from build123d import *

# Parameters (mm, degrees)
SKETCH1_W                 = 72.58
SKETCH1_H                 = 57.34
SKETCH1_R                 = 1.5
BOSS_EXTRUDE1_DEPTH       = 4.1
SKETCH2_W                 = 72.58
SKETCH2_H                 = 57.34
SKETCH2_R                 = 1.5
BOSS_EXTRUDE2_DEPTH       = 0.5
SKETCH2_4_W               = 72.58
SKETCH2_4_H               = 57.34
SKETCH2_4_R               = 1.5
BOSS_EXTRUDE3_DEPTH       = 4
BOSS_EXTRUDE4_START       = 4
BOSS_EXTRUDE4_OUTLINE_W   = 72.58
BOSS_EXTRUDE4_OUTLINE_H   = 57.34
BOSS_EXTRUDE4_OUTLINE_W_2 = 68.58
BOSS_EXTRUDE4_OUTLINE_H_2 = 53.34
BOSS_EXTRUDE4_DEPTH       = 1.5
SKETCH4_W                 = 70.58
SKETCH4_H                 = 55.34
SKETCH4_W_2               = 68.58
SKETCH4_H_2               = 53.34
BOSS_EXTRUDE5_DEPTH       = 10
FILLET1_R                 = 1
FILLET2_R                 = 0.5
FILLET3_R                 = 0.75
SKETCH3_W                 = 36.5
SKETCH3_H                 = 36.5
CUT_EXTRUDE1_DEPTH        = 51.230399162
SKETCH6_W                 = 11
SKETCH6_H                 = 12
SKETCH6_W_2               = 13.6
SKETCH6_H_2               = 13.6
CUT_EXTRUDE2_DEPTH        = 3
CHAMFER1_SIZE             = 5
SKETCH7_R                 = 3.5
SKETCH7_R_2               = 1.5
CUT_EXTRUDE3_DEPTH        = 3


# Read off the part's stored shape, not the designer's step: Boss-Extrude4
with BuildPart() as part:
    # Sketch1 → Boss-Extrude1 (new body)
    with BuildSketch(Plane(origin=(0, 0, 0), x_dir=(1, 0, 0), z_dir=(0, 1, 0))):
        Rectangle(SKETCH1_W, SKETCH1_H)
        with Locations(Location((-19.05, 24.13, 0), (0, 0, 270))):
            Circle(SKETCH1_R, mode=Mode.SUBTRACT)
        with Locations(Location((31.75, 8.89, 0), (0, 0, 270))):
            Circle(SKETCH1_R, mode=Mode.SUBTRACT)
        with Locations(Location((31.75, -19.05, 0), (0, 0, 270))):
            Circle(SKETCH1_R, mode=Mode.SUBTRACT)
        with Locations(Location((-20.32, -24.13, 0), (0, 0, 270))):
            Circle(SKETCH1_R, mode=Mode.SUBTRACT)
    extrude(amount=BOSS_EXTRUDE1_DEPTH)

    # Sketch2 → Boss-Extrude2 (add)
    with BuildSketch(Plane(origin=(0, 4.1, 0), x_dir=(1, 0, 0), z_dir=(0, 1, 0))):
        Rectangle(SKETCH2_W, SKETCH2_H)
        with BuildLine():
            Line((-31.29, -23.67), (-31.29, 23.67))
            Line((-31.29, 23.67), (-22.519639751, 23.67))
            ThreePointArc((-22.519639751, 23.67), (-19.05, 20.63), (-15.580360249, 23.67))
            Line((-15.580360249, 23.67), (31.29, 23.67))
            Line((31.29, 23.67), (31.29, 12.359639751))
            ThreePointArc((31.29, 12.359639751), (28.25, 8.89), (31.29, 5.420360249))
            Line((31.29, 5.420360249), (31.29, -15.580360249))
            ThreePointArc((31.29, -15.580360249), (28.25, -19.05), (31.29, -22.519639751))
            Line((31.29, -22.519639751), (31.29, -23.67))
            Line((31.29, -23.67), (-16.850360249, -23.67))
            ThreePointArc((-16.850360249, -23.67), (-20.32, -20.63), (-23.789639751, -23.67))
            Line((-23.789639751, -23.67), (-31.29, -23.67))
        make_face(mode=Mode.SUBTRACT)
        with Locations(Location((31.75, 8.89, 0), (0, 0, 270))):
            Circle(SKETCH2_R, mode=Mode.SUBTRACT)
        with Locations(Location((-19.05, 24.13, 0), (0, 0, 270))):
            Circle(SKETCH2_R, mode=Mode.SUBTRACT)
        with Locations(Location((-20.32, -24.13, 0), (0, 0, 270))):
            Circle(SKETCH2_R, mode=Mode.SUBTRACT)
        with Locations(Location((31.75, -19.05, 0), (0, 0, 270))):
            Circle(SKETCH2_R, mode=Mode.SUBTRACT)
    extrude(amount=BOSS_EXTRUDE2_DEPTH)

    # Sketch2<4> → Boss-Extrude3 (add)
    with BuildSketch(Plane(origin=(0, 4.1, 0), x_dir=(1, 0, 0), z_dir=(0, 1, 0))):
        Rectangle(SKETCH2_4_W, SKETCH2_4_H)
        with BuildLine():
            ThreePointArc((-21.457986711, 26.67), (-19.05, 20.63), (-16.642013289, 26.67))
            Line((-16.642013289, 26.67), (34.29, 26.67))
            Line((34.29, 26.67), (34.29, 11.297986711))
            ThreePointArc((34.29, 11.297986711), (28.25, 8.89), (34.29, 6.482013289))
            Line((34.29, 6.482013289), (34.29, -16.642013289))
            ThreePointArc((34.29, -16.642013289), (28.25, -19.05), (34.29, -21.457986711))
            Line((34.29, -21.457986711), (34.29, -26.67))
            Line((34.29, -26.67), (-17.912013289, -26.67))
            ThreePointArc((-17.912013289, -26.67), (-20.32, -20.63), (-22.727986711, -26.67))
            Line((-22.727986711, -26.67), (-34.29, -26.67))
            Line((-34.29, -26.67), (-34.29, 26.67))
            Line((-34.29, 26.67), (-21.457986711, 26.67))
        make_face(mode=Mode.SUBTRACT)
        with Locations(Location((-19.05, 24.13, 0), (0, 0, 270))):
            Circle(SKETCH2_4_R, mode=Mode.SUBTRACT)
        with Locations(Location((-20.32, -24.13, 0), (0, 0, 270))):
            Circle(SKETCH2_4_R, mode=Mode.SUBTRACT)
        with Locations(Location((31.75, -19.05, 0), (0, 0, 270))):
            Circle(SKETCH2_4_R, mode=Mode.SUBTRACT)
        with Locations(Location((31.75, 8.89, 0), (0, 0, 270))):
            Circle(SKETCH2_4_R, mode=Mode.SUBTRACT)
    extrude(amount=BOSS_EXTRUDE3_DEPTH)

    # Boss-Extrude4 outline → Boss-Extrude4 (add)
    with BuildSketch(Plane(origin=(0, 4.1, 0), x_dir=(1, 0, 0), z_dir=(0, 1, 0)).offset(BOSS_EXTRUDE4_START)):
        Rectangle(BOSS_EXTRUDE4_OUTLINE_W, BOSS_EXTRUDE4_OUTLINE_H)
        Rectangle(BOSS_EXTRUDE4_OUTLINE_W_2, BOSS_EXTRUDE4_OUTLINE_H_2, mode=Mode.SUBTRACT)
    extrude(amount=BOSS_EXTRUDE4_DEPTH)

    # Sketch4 → Boss-Extrude5 (add)
    with BuildSketch(Plane(origin=(0, 9.6, 0), x_dir=(1, 0, 0), z_dir=(0, 1, 0))):
        Rectangle(SKETCH4_W, SKETCH4_H)
        Rectangle(SKETCH4_W_2, SKETCH4_H_2, mode=Mode.SUBTRACT)
    extrude(amount=BOSS_EXTRUDE5_DEPTH)

    # Fillet1
    fillet1_edges = [part.edges().sort_by_distance(p)[0] for p in [
        (36.29, 4.8, -28.67),
        (36.29, 4.8, 28.67),
        (-36.29, 4.8, 28.67),
        (-36.29, 4.8, -28.67),
    ]]
    fillet(fillet1_edges, radius=FILLET1_R)

    # Fillet2
    fillet2_edges = [part.edges().sort_by_distance(p)[0] for p in [
        (34.29, 12.1, 26.67),
        (-34.29, 12.1, 26.67),
        (-34.29, 12.1, -26.67),
        (34.29, 12.1, -26.67),
    ]]
    fillet(fillet2_edges, radius=FILLET2_R)

    # Fillet3
    # the kernel refuses this fillet: 0.75 mm, written as the material it adds along each edge
    with BuildSketch(Plane(origin=(-17.912013289, 0.983317982, 26.67), x_dir=(1, 0, 0), z_dir=(0, 1, 0)), Plane(origin=(-21.457986711, 0.983317982, -26.67), x_dir=(-1, 0, 0), z_dir=(0, 1, 0)), Plane(origin=(34.29, 0.983317982, -11.297986711), x_dir=(0, 0, -1), z_dir=(0, 1, 0)), Plane(origin=(34.29, 0.983317982, 16.642013289), x_dir=(0, 0, -1), z_dir=(0, 1, 0))) as fillet3_piece_1:
        with BuildLine():
            CenterArc((1.446672807, 0.75), FILLET3_R, 155.091114703, 114.908885297)
            ThreePointArc((0.766438775, 1.065882353), (0.433642713, 0.496683524), (0, 0))
            Line((0, 0), (1.446672807, 0))
        make_face()
    extrude(amount=7.116682018)
    with BuildSketch(Plane(origin=(-22.727986711, 0.983317982, 26.67), x_dir=(-1, 0, 0), z_dir=(0, 1, 0)), Plane(origin=(-16.642013289, 0.983317982, -26.67), x_dir=(1, 0, 0), z_dir=(0, 1, 0)), Plane(origin=(34.29, 0.983317982, -6.482013289), x_dir=(0, 0, 1), z_dir=(0, 1, 0)), Plane(origin=(34.29, 0.983317982, 21.457986711), x_dir=(0, 0, 1), z_dir=(0, 1, 0))) as fillet3_piece_2:
        with BuildLine():
            CenterArc((1.446672807, -0.75), FILLET3_R, 90, 114.908885297)
            ThreePointArc((0.766438775, -1.065882353), (0.433642713, -0.496683524), (0, 0))
            Line((0, 0), (1.446672807, 0))
        make_face()
    extrude(amount=7.116682018)
    with BuildSketch(Plane(origin=(31.29, 2.225, -23.67), x_dir=(-1, 0, 0), z_dir=(0, 1, 0)), Plane(origin=(31.29, 2.225, 23.67), x_dir=(0, 0, -1), z_dir=(0, 1, 0)), Plane(origin=(-31.29, 2.225, 23.67), x_dir=(1, 0, 0), z_dir=(0, 1, 0)), Plane(origin=(-31.29, 2.225, -23.67), x_dir=(0, 0, 1), z_dir=(0, 1, 0))) as fillet3_piece_3:
        with BuildLine():
            CenterArc((FILLET3_R, FILLET3_R), FILLET3_R, 180, 90)
            Line((0, FILLET3_R), (0, 0))
            Line((0, 0), (FILLET3_R, 0))
        make_face()
    extrude(amount=2.375)
    with BuildSketch(Plane(origin=(31.29, 2.588815876, -12.359639751), x_dir=(-0.977977776437884, 0, 0.20870905297473832), z_dir=(0, 1, 0)), Plane(origin=(31.29, 2.588815876, 15.580360249), x_dir=(-0.9779777764378829, 0, 0.2087090529747441), z_dir=(0, 1, 0)), Plane(origin=(-16.850360249, 2.588815876, 23.67), x_dir=(-0.2087090529747233, 0, -0.9779777764378872), z_dir=(0, 1, 0)), Plane(origin=(-22.519639751, 2.588815876, -23.67), x_dir=(0.20870905297473083, 0, 0.9779777764378856), z_dir=(0, 1, 0))) as fillet3_piece_4:
        with BuildLine():
            CenterArc((0.607324209, -0.747693586), FILLET3_R, 94.494558388, 73.458731432)
            Line((-0.126159123, -0.591161796), (0, 0))
            ThreePointArc((0, 0), (0.274275449, -0.010763267), (0.548550899, 0))
        make_face()
    extrude(amount=2.011184124)
    with BuildSketch(Plane(origin=(31.29, 2.588815876, -5.420360249), x_dir=(-0.9779777764378846, 0, -0.20870905297473547), z_dir=(0, 1, 0)), Plane(origin=(31.29, 2.588815876, 22.519639751), x_dir=(-0.9779777764378821, 0, -0.20870905297474715), z_dir=(0, 1, 0)), Plane(origin=(-23.789639751, 2.588815876, 23.67), x_dir=(0.20870905297472817, 0, -0.9779777764378861), z_dir=(0, 1, 0)), Plane(origin=(-15.580360249, 2.588815876, -23.67), x_dir=(-0.2087090529747233, 0, 0.9779777764378872), z_dir=(0, 1, 0))) as fillet3_piece_5:
        with BuildLine():
            CenterArc((0.607324209, 0.747693586), FILLET3_R, 192.04671018, 73.458731432)
            Line((-0.126159123, 0.591161796), (0, 0))
            ThreePointArc((0, 0), (0.274275449, 0.010763267), (0.548550899, 0))
        make_face()
    extrude(amount=2.011184124)

    # Sketch3 → Cut-Extrude1 (cut, through all)
    with BuildSketch(Plane(origin=(0, 0, 0), x_dir=(1, 0, 0), z_dir=(0, 1, 0))):
        Rectangle(SKETCH3_W, SKETCH3_H)
    extrude(amount=CUT_EXTRUDE1_DEPTH, mode=Mode.SUBTRACT)

    # Sketch6 → Cut-Extrude2 (cut)
    with BuildSketch(Plane.ZY.offset(35.29)):
        with Locations((19.52, 15.6)):
            Rectangle(SKETCH6_W, SKETCH6_H)
        with Locations((-11.29, 16.4)):
            Rectangle(SKETCH6_W_2, SKETCH6_H_2)
    extrude(amount=-CUT_EXTRUDE2_DEPTH, mode=Mode.SUBTRACT)

    # Chamfer1
    chamfer1_edges = [part.edges().sort_by_distance(p)[0] for p in [
        (18.25, 2.05, 18.25),
        (18.25, 2.05, -18.25),
        (-18.25, 2.05, -18.25),
        (-18.25, 2.05, 18.25),
    ]]
    chamfer(chamfer1_edges, length=CHAMFER1_SIZE)

    # Sketch7 → Cut-Extrude3 (cut)
    # profile 1 of 4: a face of its own
    with BuildSketch(Plane.XZ):
        with Locations(Location((-20.32, 24.13, 0), (0, 0, 270))):
            Circle(SKETCH7_R)
        with Locations(Location((-20.32, 24.13, 0), (0, 0, 270))):
            Circle(SKETCH7_R_2, mode=Mode.SUBTRACT)
    # profile 2 of 4: a face of its own
    with BuildSketch(Plane.XZ):
        with Locations(Location((-19.05, -24.13, 0), (0, 0, 270))):
            Circle(SKETCH7_R)
        with Locations(Location((-19.05, -24.13, 0), (0, 0, 270))):
            Circle(SKETCH7_R_2, mode=Mode.SUBTRACT)
    # profile 3 of 4: a face of its own
    with BuildSketch(Plane.XZ):
        with Locations(Location((31.75, -8.89, 0), (0, 0, 270))):
            Circle(SKETCH7_R)
        with Locations(Location((31.75, -8.89, 0), (0, 0, 270))):
            Circle(SKETCH7_R_2, mode=Mode.SUBTRACT)
    # profile 4 of 4: a face of its own
    with BuildSketch(Plane.XZ):
        with Locations(Location((31.75, 19.05, 0), (0, 0, 270))):
            Circle(SKETCH7_R)
        with Locations(Location((31.75, 19.05, 0), (0, 0, 270))):
            Circle(SKETCH7_R_2, mode=Mode.SUBTRACT)
    extrude(amount=-CUT_EXTRUDE3_DEPTH, mode=Mode.SUBTRACT)


solid = part.part
Can you work these out from the model? Positions are in its coordinate system, mm. A direction names the side the tool comes from. Round coordinates to 2 decimals unless told otherwise and drop trailing zeros. Order: outer loops, then holes, each group sorted by start corner. A loop starts at its lowest first (then second) coordinate and runs counter-clockwise, first axis right, second up. Notation, with made-up numbers: M 0.25,13.5 L 31.25,13.5 A14 ccw 31.25,38.5 Z; hole C 57.25,-10 d7. An arc over 180 degrees is marked long. Use a Markdown table: item, result.
1) If we mould it in two halves opening along X, with no side actions, what happens to faces 1 (the face through (0, 2, -18.25)), 2 (the face through (35.29, 15, 0)), 3 (the face through (0, 15, 27.67))? For each: +X half, -X half, draft (parallel to the pull), parting line (faces both ways), or undercut.
Geometry says:
| item | result |
|---|---|
| face 1 | undercut |
| face 2 | +X half |
| face 3 | draft |
2) Imagine slicing it at B-B (x = -8). List the corners of the cut face in (y, z) for me.
Geometry says:
| item | result |
|---|---|
| outline | M 0,-28.67 L 9.6,-28.67 L 9.6,-27.67 L 19.6,-27.67 L 19.6,-26.67 L 4.6,-26.67 L 4.6,-23.67 L 4.1,-23.67 L 4.1,-18.25 L 0,-18.25 Z; M 0,18.25 L 4.1,18.25 L 4.1,23.67 L 4.6,23.67 L 4.6,26.67 L 19.6,26.67 L 19.6,27.67 L 9.6,27.67 L 9.6,28.67 L 0,28.67 Z |
3) Imagine slicing it at D-D (z = -8.89). List the corners of the cut face in (x, y) for me, then the cut area to 3 significant figures.
Geometry says:
| item | result |
|---|---|
| outline | M -36.29,0 L -18.25,0 L -18.25,4.1 L -31.29,4.1 L -31.29,4.6 L -34.29,4.6 L -34.29,9.6 L -36.29,9.6 Z; M 18.25,0 L 28.25,0 L 28.25,3 L 30.25,3 L 30.25,8.1 L 28.25,8.1 L 28.25,4.1 L 18.25,4.1 Z; M 33.25,3 L 35.25,3 L 35.25,0 L 36.29,0 L 36.29,9.6 L 35.29,9.6 L 35.29,19.6 L 34.29,19.6 L 34.29,8.1 L 33.25,8.1 Z |
| area | 169 mm² |
4) If I drill on line 1 along X through (y, z) = (2, -8.89); line 2 along Z through (x, y) = (31.75, 4.65); line 3 along Z through (x, y) = (-0.5, 7.5), over which ranges is the centre line in solid material (lowest first)?
Geometry says:
| item | result |
|---|---|
| line 1 | x = -36.29 to -18.25, 18.25 to 28.25, 35.25 to 36.29 |
| line 2 | z = -28.67 to -26.67, -12.39 to -10.39, -7.39 to -5.39, 15.55 to 17.55, 20.55 to 22.55, 26.67 to 28.67 |
| line 3 | z = -28.67 to -26.67, 26.67 to 28.67 |
5) I'm going to push flat-ended pins straight in: P1, Ø3, axis at x = -28.5, z = -20.5, coming from the +Y side; P2, Ø1.1, axis at x = -34.5, y = 15.5, coming from the +Z side; P3, Ø2.5, axis at x = -19.05, z = -24.13, coming from the -Y side; P4, Ø8, axis at x = 12, y = 13, coming from the -Z side. Where does each tip first touch, or does it pass through?
Geometry says:
| item | result |
|---|---|
| P1 | stops at y = 4.1 |
| P2 | stops at z = 27.67 |
| P3 | passes through |
| P4 | stops at z = -28.67 |
6) Imagine slicing it at A-A (y = 18). List the corners of the cut face in (x, z) for me, then the cut area to 3 significant figures.
Geometry says:
| item | result |
|---|---|
| outline | M -35.29,-27.67 L 35.29,-27.67 L 35.29,27.67 L -35.29,27.67 L -35.29,25.02 L -34.29,25.02 L -34.29,26.17 A0.5 cw -33.79,26.67 L 33.79,26.67 A0.5 cw 34.29,26.17 L 34.29,-26.17 A0.5 cw 33.79,-26.67 L -33.79,-26.67 A0.5 cw -34.29,-26.17 L -34.29,-18.09 L -35.29,-18.09 Z; M -35.29,-4.49 L -34.29,-4.49 L -34.29,14.02 L -35.29,14.02 Z |
| area | 223 mm² |
7) On a 3-axis mill with a long thin cutter (end or side, diameter ignored), from which of +Z, -Z, +X, -X, +Y, -Y can I reach the whole of each face in a straight line? I mean faces 4 (the face through (30, 3, -9)), 5 (the face through (28.25, 6.07, -8.99)), 6 (the face through (-15.7, 2, 15.8)). Say none if no direction works.
Geometry says:
| item | result |
|---|---|
| face 4 | -Y |
| face 5 | +Y |
| face 6 | +Y, -Y |
8) Imagine slicing it at C-C (z = -15). List the corners of the cut face in (x, y) for me, then the cut area to 3 significant figures.
Geometry says:
| item | result |
|---|---|
| outline | M -36.29,0 L -16.5,0 L -16.5,4.1 L -31.29,4.1 L -31.29,4.6 L -34.29,4.6 L -34.29,9.6 L -36.29,9.6 Z; M 16.5,0 L 36.29,0 L 36.29,9.6 L 35.29,9.6 L 35.29,19.6 L 34.29,19.6 L 34.29,4.6 L 31.29,4.6 L 31.29,4.1 L 16.5,4.1 Z |
| area | 197 mm² |
